Input: part model. Units: mm. Frame: model coordinates. Face numbers are marked on the shaded views. A direction names the side the tool comes from. Give positions to 0.01 mm unless a question says otherwise; leave off trailing zeros. Order: outer loops, then holes, each group sorted by start corner. A loop starts at its lowest first (then second) coordinate and runs counter-clockwise, first axis right, second up. Notation, with made-up numbers: (78.5, 26.25) - (130.5, 26.25) arc R33 cw to (130.5, 56.25) - close; hole circle Ø9 at (5, 53). An arc over 180 degrees is marked (long way). Answer in a Markdown table with one row per item. Add a question column.
1. Section query C-C on z = 0.25. Return loops of the section in (x, y).
2. Contact query for flat-ended pins moving along their axis: pin 1 (0.8 mm diameter, centred on x = -0.5, z = 2, fed in from +Y); pin 2 (1 mm diameter, centred on y = -1.5, z = -3.5, fed in from -X); pin 3 (1.1 mm diameter, centred on x = -1.5, z = 2, fed in from -Y). Output: stop coordinate, or through.
3. Access query for the marked faces 1, 2 and 3. Directions: +Z, -Z, +X, -X, +Y, -Y. A direction counts if a zero-diameter tool reaches every point of the face in a straight line with its end or side. Return the directions, or none.
4. Mould query, pull axis Y, two halves, no side actions, for the marked faces 4, 5 and 6. Classes: released by +Y, released by -Y, zero draft, split by the parting line, or undercut.
5. Section query A-A on y = 0. Return loops of the section in (x, z), and give its area (3 significant figures).
6. Section query D-D on z = -3. Return loops of the section in (x, y), and give its area (3 significant figures).
7. Ray query, line 1 (Z direction, x = 1.1, y = 1.7); line 2 (Z direction, x = 0.55, y = 1.65); line 3 (X direction, y = -2.25, z = 0.25). Return the intervals inside material, ascending. Write a range as [from, to].
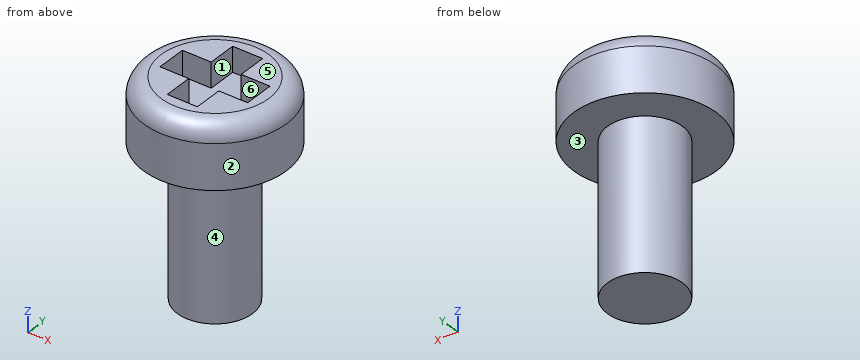
```python
from build123d import *

# Parameters (mm, degrees)
SKETCH_R     = 2.85
PAD_DEPTH    = 2.5
POCKET_DEPTH = 1
FILLET_R     = 0.7
SKETCH002_R  = 1.5
PAD001_DEPTH = 6


with BuildPart() as part:
    # Sketch → Pad (new body)
    with BuildSketch(Plane.XY):
        Circle(SKETCH_R)
    extrude(amount=PAD_DEPTH)

    # Sketch001 (on Face3 of Pad) → Pocket (cut)
    with BuildSketch(Plane.XY.offset(2.5)):
        Polygon((-0.6, 1.75), (0.6, 1.75), (0.6, 0.6), (1.75, 0.6), (1.75, -0.6), (0.6, -0.6), (0.6, -1.75), (-0.6, -1.75), (-0.6, -0.6), (-1.75, -0.6), (-1.75, 0.6), (-0.6, 0.6), align=None)
    extrude(amount=-POCKET_DEPTH, mode=Mode.SUBTRACT)

    # Fillet
    fillet_edges = [part.edges().sort_by_distance(p)[0] for p in [
        (-2.85, 0, 2.5),
    ]]
    fillet(fillet_edges, radius=FILLET_R)

    # Sketch002 (on Face3 of Fillet) → Pad001 (join)
    with BuildSketch(Plane(origin=(0, 0, 0), x_dir=(1, 0, 0), z_dir=(0, 0, -1))):
        Circle(SKETCH002_R)
    extrude(amount=PAD001_DEPTH)


solid = part.part
```
Answer:
| question | item | result |
|---|---|---|
| 1 | outline | circle Ø5.7 at (0, 0) |
| 2 | pin 1 | stops at y = 2.85 |
| 2 | pin 2 | stops at x = -1.12 |
| 2 | pin 3 | stops at y = -2.68 |
| 3 | face 1 | +Z |
| 3 | face 2 | +Z, -Z |
| 3 | face 3 | -Z |
| 4 | face 4 | split by the parting line |
| 4 | face 5 | zero draft |
| 4 | face 6 | undercut |
| 5 | outline | (-2.85, 0) - (-1.5, 0) - (-1.5, -6) - (1.5, -6) - (1.5, 0) - (2.85, 0) - (2.85, 1.8) arc R0.7 ccw to (2.15, 2.5) - (1.75, 2.5) - (1.75, 1.5) - (-1.75, 1.5) - (-1.75, 2.5) - (-2.15, 2.5) arc R0.7 ccw to (-2.85, 1.8) - close |
| 5 | area | 28.5 mm² |
| 6 | outline | circle Ø3 at (0, 0) |
| 6 | area | 7.07 mm² |
| 7 | line 1 | z = [0, 2.5] |
| 7 | line 2 | z = [0, 1.5] |
| 7 | line 3 | x = [-1.75, 1.75] |
